Verification items for the finished model (mm, model axes). Face numbers are marked on the shaded views. Give positions to 0.01 mm unless a question says otherwise; leave off trailing zeros. Write each loop counter-clockwise with the first axis right and the second up, starting at its lowest first coordinate (ties: lowest second). Pieces come first, ordered by that corner, then holes. Notation, with made-up numbers: M 89,55.5 L 93,55.5 A14 ccw 93,64.5 Z; hole C 34,63 d8. An arc over 180 degrees is marked long. Write item = value, one per line.
from build123d import *

# Parameters (mm, degrees)
SKETCH_1_R      = 26
EXTRUDE_1_DEPTH = 10
SKETCH_2_R      = 26
SKETCH_2_R_2    = 1.5
EXTRUDE_2_DEPTH = 3
FILLET_1_R      = 4
FILLET_2_R      = 4


with BuildPart() as part:
    # 草图1 → 凸台-拉伸1 (new body)
    with BuildSketch(Plane.XY):
        Circle(SKETCH_1_R)
        with BuildLine():
            ThreePointArc((3, -21), (0, -24), (-3, -21))
            Line((-3, -21), (-3, -17.088665834))
            ThreePointArc((-3, -17.088665834), (-8.675, -15.025540756), (-13.299218729, -11.142409129))
            Line((-13.299218729, -11.142409129), (-16.686533479, -13.098076211))
            ThreePointArc((-16.686533479, -13.098076211), (-20.784609691, -12), (-19.686533479, -7.901923789))
            Line((-19.686533479, -7.901923789), (-16.299218729, -5.946256706))
            ThreePointArc((-16.299218729, -5.946256706), (-17.35, 0), (-16.299218729, 5.946256706))
            Line((-16.299218729, 5.946256706), (-19.686533479, 7.901923789))
            ThreePointArc((-19.686533479, 7.901923789), (-20.784609691, 12), (-16.686533479, 13.098076211))
            Line((-16.686533479, 13.098076211), (-13.299218729, 11.142409129))
            ThreePointArc((-13.299218729, 11.142409129), (-8.675, 15.025540756), (-3, 17.088665834))
            Line((-3, 17.088665834), (-3, 21))
            ThreePointArc((-3, 21), (0, 24), (3, 21))
            Line((3, 21), (3, 17.088665834))
            ThreePointArc((3, 17.088665834), (8.675, 15.025540756), (13.299218729, 11.142409129))
            Line((13.299218729, 11.142409129), (16.686533479, 13.098076211))
            ThreePointArc((16.686533479, 13.098076211), (20.784609691, 12), (19.686533479, 7.901923789))
            Line((19.686533479, 7.901923789), (16.299218729, 5.946256706))
            ThreePointArc((16.299218729, 5.946256706), (17.085285262, 3.019193191), (17.35, 0))
            ThreePointArc((17.35, 0), (17.085285262, -3.019193191), (16.299218729, -5.946256706))
            Line((16.299218729, -5.946256706), (19.686533479, -7.901923789))
            ThreePointArc((19.686533479, -7.901923789), (20.784609691, -12), (16.686533479, -13.098076211))
            Line((16.686533479, -13.098076211), (13.299218729, -11.142409129))
            ThreePointArc((13.299218729, -11.142409129), (8.675, -15.025540756), (3, -17.088665834))
            Line((3, -17.088665834), (3, -21))
        make_face(mode=Mode.SUBTRACT)
    extrude(amount=EXTRUDE_1_DEPTH)

    # 草图2 → 凸台-拉伸2 (add)
    with BuildSketch(Plane.XY.offset(10)):
        Circle(SKETCH_2_R)
        with Locations((0, 14.93)):
            Circle(SKETCH_2_R_2, mode=Mode.SUBTRACT)
        with Locations((12.929759279, 7.465)):
            Circle(SKETCH_2_R_2, mode=Mode.SUBTRACT)
        with Locations((12.929759279, -7.465)):
            Circle(SKETCH_2_R_2, mode=Mode.SUBTRACT)
        with Locations((0, -14.93)):
            Circle(SKETCH_2_R_2, mode=Mode.SUBTRACT)
        with Locations((-12.929759279, -7.465)):
            Circle(SKETCH_2_R_2, mode=Mode.SUBTRACT)
        with Locations((-12.929759279, 7.465)):
            Circle(SKETCH_2_R_2, mode=Mode.SUBTRACT)
        Circle(SKETCH_2_R_2, mode=Mode.SUBTRACT)
    extrude(amount=EXTRUDE_2_DEPTH)

    # 圆角1
    # the kernel refuses this fillet: 4 mm, written as the material it takes off along each edge
    with BuildSketch(Plane(origin=(0, 0, 0), x_dir=(1, 0, 0), z_dir=(0, -1, 0))) as fillet_1_piece_1:
        with BuildLine():
            CenterArc((26 - FILLET_1_R, FILLET_1_R), FILLET_1_R, 270, 90)
            Line((26 - FILLET_1_R, 0), (26, 0))
            Line((26, 0), (26, FILLET_1_R))
        make_face()
    revolve(axis=Axis((0, 0, 0), (0, 0, 1)), mode=Mode.SUBTRACT)
    with BuildSketch(Plane(origin=(0, 0, 13), x_dir=(1, 0, 0), z_dir=(0, -1, 0))) as fillet_1_piece_2:
        with BuildLine():
            CenterArc((26 - FILLET_1_R, -FILLET_1_R), FILLET_1_R, 0, 90)
            Line((26 - FILLET_1_R, 0), (26, 0))
            Line((26, 0), (26, -FILLET_1_R))
        make_face()
    revolve(axis=Axis((0, 0, 13), (0, 0, 1)), mode=Mode.SUBTRACT)

    # 圆角2
    fillet_2_edges = [part.edges().sort_by_distance(p)[0] for p in [
        (-17.35, 0, 0),
        (-8.675, 15.025540756, 0),
        (8.675, 15.025540756, 0),
        (17.35, 0, 0),
        (8.675, -15.025540756, 0),
        (-8.675, -15.025540756, 0),
    ]]
    fillet(fillet_2_edges, radius=FILLET_2_R)


solid = part.part
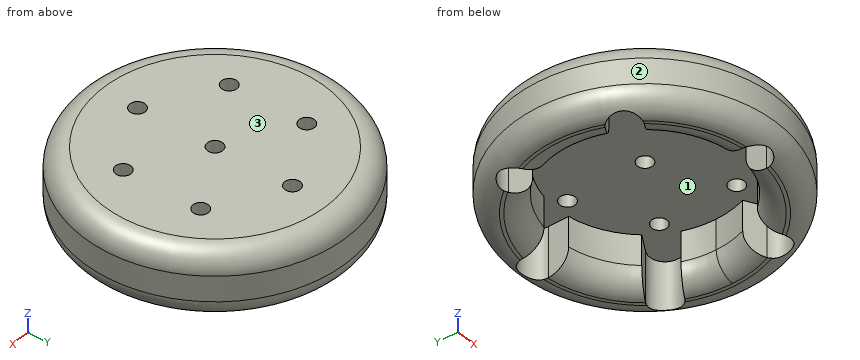
1) Cross-section at A-A on x = 0. Record the boundary of the cut face in (y, z), plus the area to 3 significant figures.
From the geometry:
outline = M -26,4 A4 ccw -24,0.54 L -24,10 L -16.43,10 L -16.43,13 L -22,13 A4 ccw -26,9 Z; M -13.43,10 L -1.5,10 L -1.5,13 L -13.43,13 Z; M 1.5,10 L 13.43,10 L 13.43,13 L 1.5,13 Z; M 16.43,10 L 24,10 L 24,0.54 A4 ccw 26,4 L 26,9 A4 ccw 22,13 L 16.43,13 Z
area = 156 mm^2
2) Material ranges on probe 1 along Y at (x, z) = (0, 11.9) (3 decimals); probe 2 along Y at (x, z) = (0, 12.4); probe 3 along Y at (x, z) = (19.5, 2), recorded low to high. Write a range as from..to.
From the geometry:
probe_1 = -24.755..-16.43, -13.43..-1.5, 1.5..13.43, 16.43..24.755
probe_2 = -24.11..-16.43, -13.43..-1.5, 1.5..13.43, 16.43..24.11
probe_3 = -16.38..-13.2, -7.79..7.79, 13.2..16.38
3) Cross-section at B-B on z = 2.75. Record the boundary of the cut face in (x, y).
From the geometry:
outline = C 0,0 d51.6; hole M -19.69,-7.9 A3 ccw -16.69,-13.1 L -13.48,-11.24 A17.55 ccw -3,-17.29 L -3,-21 A3 ccw 3,-21 L 3,-17.29 A17.55 ccw 13.48,-11.24 L 16.69,-13.1 A3 ccw 19.69,-7.9 L 16.48,-6.05 A17.55 ccw 16.48,6.05 L 19.69,7.9 A3 ccw 16.69,13.1 L 13.48,11.24 A17.55 ccw 3,17.29 L 3,21 A3 ccw -3,21 L -3,17.29 A17.55 ccw -13.48,11.24 L -16.69,13.1 A3 ccw -19.69,7.9 L -16.48,6.05 A17.55 ccw -16.48,-6.05 Z
4) Draft check along Y on the marked faces 1, 2 and 3. Enter one of: +Y half, -Y half, draft (parallel to the pull), parting line (faces both ways), or undercut.
From the geometry:
face_1 = undercut
face_2 = parting line
face_3 = draft
5) Depth check by flat-ended pin: P1, Ø5, axis at x = 0, y = -12.5, coming from the -Z side; P2, Ø4, axis at x = -12.93, y = -7.46, coming from the +Z side; P3, Ø4.5, axis at y = -18.5, z = 3.5, coming from the -X side; P4, Ø1.2, axis at y = 19, z = 4.5, coming from the +X side. Enter the tip coordinate at first touch or a pass-through.
From the geometry:
P1 = 10
P2 = 13
P3 = -20.28
P4 = 18.37
